Check sheet for the modelled part. Datum: model origin and axes. Units: mm. A direction names the side the tool comes from. Give positions to 0.01 mm unless a question says otherwise; leave off trailing zeros. Order: outer loops, then holes, each group sorted by start corner. A loop starts at its lowest first (then second) coordinate and runs counter-clockwise, first axis right, second up.
```python
from build123d import *

# Parameters (mm, degrees)
SKETCH_1_R          = 6
EXTRUDE_1_DEPTH     = 250
CUT_EXTRUDE_START   = -5.8
SKETCH_2_R          = 6
SKETCH_2_R_2        = 5
CUT_EXTRUDE_1_DEPTH = 5.8


with BuildPart() as part:
    # ｽｹｯﾁ1 → ﾎﾞｽ - 押し出し1 (new body)
    with BuildSketch(Plane.XY):
        Circle(SKETCH_1_R)
    extrude(amount=EXTRUDE_1_DEPTH)

    # ｽｹｯﾁ2 → ｶｯﾄ - 押し出し1 (cut)
    with BuildSketch(Plane.XY.offset(250).offset(CUT_EXTRUDE_START)):
        Circle(SKETCH_2_R)
        Circle(SKETCH_2_R_2, mode=Mode.SUBTRACT)
    cut_extrude_1 = extrude(amount=CUT_EXTRUDE_1_DEPTH, mode=Mode.SUBTRACT)

    # ﾐﾗｰ1: ｶｯﾄ - 押し出し1 across plane
    add(cut_extrude_1.mirror(Plane.XY.offset(125)), mode=Mode.SUBTRACT)


solid = part.part
```
(1) Cross-section at B-B on z = 175. Enter the section's corners in (x, y).
Response values:
outline: circle Ø12 at (0, 0)
(2) Cross-section at A-A on x = 2. Enter the section's corners in (y, z), then the cut area to 3 significant figures.
Response values:
outline: (-5.66, 5.8) - (-4.58, 5.8) - (-4.58, 0) - (4.58, 0) - (4.58, 5.8) - (5.66, 5.8) - (5.66, 244.2) - (4.58, 244.2) - (4.58, 250) - (-4.58, 250) - (-4.58, 244.2) - (-5.66, 244.2) - close
area: 2,800 mm2
(3) Material ranges on L1, parallel to X at y = 0.5, z = 116; L2, parallel to Y at x = 0.75, z = 81; L3, parallel to Z at x = 5.5, y = 0, recorded low to high.
Response values:
L1: x = -5.98 to 5.98
L2: y = -5.95 to 5.95
L3: z = 5.8 to 244.2
(4) Gauge pin test, flat ends, axial feed: pin 1 Ø1.5 at (x, z) = (3.5, 92) entering from -Y; pin 2 Ø3 at (x, z) = (3.5, 186) entering from -Y; pin 3 Ø6 at (y, z) = (4, 106) entering from -X. Record the tip position at first contact, or that the pin passes through.
Response values:
pin 1: stops at y = -5.33
pin 2: stops at y = -5.66
pin 3: stops at x = -5.92
(5) Set-up check for faces 1 (the face through (-6, 0, 123)), 2 (the face through (-4, 4, 244.2)), 3 (the face through (-4, 4, 5.8)): record each of +Z, -Z, +X, -X, +Y, -Y from which the full face is reachable in a straight line by a thin tool's end or side.
Response values:
face 1: +Z, -Z
face 2: +Z
face 3: -Z
